Work out the finished part from the listing and answer in its coordinate system (mm). Coordinates: 2 decimals unless noted, no trailing zeros. Write each loop counter-clockwise with the first axis right and the second up, starting at its lowest first coordinate (ties: lowest second). Pieces come first, ordered by that corner, then holes. Notation, with made-up numbers: (17, 51) - (31, 51) arc R21 cw to (31, 63) - close; hole circle Ø9 at (86, -13). An arc over 180 degrees is marked (long way). Use a Markdown table: item, result. Add a question column.
(1) The part is cut by section A-A, the plane y = 22.5. Give the vertices of the cut face in (x, z), then the cut area to 3 significant figures.
(2) Given pin 1 Ø12 at (x, y) = (153, 104) entering from +Z; pin 2 Ø1 at (x, z) = (5.5, 1.5) entering from -Y; pin 3 Ø1 at (x, z) = (172, 1) entering from +Y; pin 4 Ø0.6 at (x, z) = (196, 1) entering from -Y, each flat-ended and moving along its own axis, determine where each tip first touches the part or whether it passes through.
(3) Find the intervals of material crossed by line 1 (X direction, y = 117, z = 0.25); line 2 (X direction, y = 87, z = 1.05); line 3 (X direction, y = 84, z = 1.2), in increasing order. Write a range as from..to.
(4) The part is cut by section B-B, the plane x = 110. Give the vertices of the cut face in (y, z), then the cut area to 3 significant figures.
from build123d import *

# Parameters (mm, degrees)
SKETCH1_W               = 194
SKETCH1_H               = 227
BOSS_EXTRUDE1_DEPTH     = 2
SKETCH2_W               = 2
SKETCH2_H               = 10
BOSS_EXTRUDE2_DEPTH     = 3
LPATTERN1_COUNT         = 11
LPATTERN1_PITCH         = 20
SKETCH4_W               = 2
SKETCH4_H               = 10
BOSS_EXTRUDE3_DEPTH     = 3
LPATTERN2_COUNT         = 11
LPATTERN2_PITCH         = 20
SKETCH5_W               = 10
SKETCH5_H               = 2
BOSS_EXTRUDE4_DEPTH     = 3
LPATTERN3_COUNT         = 9
LPATTERN3_PITCH         = 20
SKETCH6_W               = 10
SKETCH6_H               = 2
BOSS_EXTRUDE5_DEPTH     = 3
LPATTERN4_COUNT         = 9
LPATTERN4_PITCH         = 20
SKETCH7_W               = 30
SKETCH7_H               = 211
CUT_EXTRUDE1_DEPTH      = 3
SKETCH8_R               = 1.75
SKETCH8_W               = 30
SKETCH8_H               = 211
CUT_EXTRUDE2_DEPTH      = 3
ENL_V_START             = -2
ESQUISSE1_W             = 1
ESQUISSE1_H             = 231.630862985
ENL_V_MAT_EXTRU_1_DEPTH = 2
ESQUISSE2_W             = 1
ESQUISSE2_H             = 7
ESQUISSE2_H_2           = 10
ESQUISSE2_W_2           = 10
ESQUISSE2_H_3           = 1
ESQUISSE2_W_3           = 14
BOSS_EXTRU_1_DEPTH      = 2
ESQUISSE3_R             = 1.75
ENL_V_MAT_EXTRU_2_DEPTH = 3


with BuildPart() as part:
    # Sketch1 → Boss-Extrude1 (new body)
    with BuildSketch(Plane.XY):
        with Locations((97, 113.5)):
            Rectangle(SKETCH1_W, SKETCH1_H)
    extrude(amount=BOSS_EXTRUDE1_DEPTH)

    # Sketch2 → Boss-Extrude2 (add)
    with BuildSketch(Plane(origin=(194, 0, 0), x_dir=(0, 0, -1), z_dir=(1, 0, 0))):
        with Locations((-1, 15)):
            Rectangle(SKETCH2_W, SKETCH2_H)
    boss_extrude2 = extrude(amount=BOSS_EXTRUDE2_DEPTH)

    # LPattern1: Boss-Extrude2 ×11
    with Locations(*[(0, i * LPATTERN1_PITCH, 0) for i in range(1, LPATTERN1_COUNT)]):
        add(boss_extrude2)

    # Sketch4 → Boss-Extrude3 (add)
    with BuildSketch(Plane.ZY):
        with Locations((1, 15)):
            Rectangle(SKETCH4_W, SKETCH4_H)
    boss_extrude3 = extrude(amount=BOSS_EXTRUDE3_DEPTH)

    # LPattern2: Boss-Extrude3 ×11
    with Locations(*[(0, i * LPATTERN2_PITCH, 0) for i in range(1, LPATTERN2_COUNT)]):
        add(boss_extrude3)

    # Sketch5 → Boss-Extrude4 (add)
    with BuildSketch(Plane.XZ):
        with Locations((179, 1)):
            Rectangle(SKETCH5_W, SKETCH5_H)
    boss_extrude4 = extrude(amount=BOSS_EXTRUDE4_DEPTH)

    # LPattern3: Boss-Extrude4 ×9
    with Locations(*[(-i * LPATTERN3_PITCH, 0, 0) for i in range(1, LPATTERN3_COUNT)]):
        add(boss_extrude4)

    # Sketch6 → Boss-Extrude5 (add)
    with BuildSketch(Plane(origin=(0, 227, 0), x_dir=(1, 0, 0), z_dir=(0, 1, 0))):
        with Locations((179, -1)):
            Rectangle(SKETCH6_W, SKETCH6_H)
    boss_extrude5 = extrude(amount=BOSS_EXTRUDE5_DEPTH)

    # LPattern4: Boss-Extrude5 ×9
    with Locations(*[(-i * LPATTERN4_PITCH, 0, 0) for i in range(1, LPATTERN4_COUNT)]):
        add(boss_extrude5)

    # Sketch7 → Cut-Extrude1 (cut, through all)
    with BuildSketch(Plane.XY.offset(2)):
        with Locations((27, 113.5)):
            Rectangle(SKETCH7_W, SKETCH7_H)
    extrude(amount=-CUT_EXTRUDE1_DEPTH, mode=Mode.SUBTRACT)

    # Sketch8 → Cut-Extrude2 (cut, through all)
    with BuildSketch(Plane.XY.offset(2)):
        with Locations((143, 15)):
            Circle(SKETCH8_R)
        with Locations((51.5, 15)):
            Circle(SKETCH8_R)
        with Locations((143, 87)):
            Circle(SKETCH8_R)
        with Locations((51.5, 87)):
            Circle(SKETCH8_R)
        with Locations((134, 112)):
            Circle(SKETCH8_R)
        with Locations((76, 112)):
            Circle(SKETCH8_R)
        with Locations((134, 161)):
            Circle(SKETCH8_R)
        with Locations((76, 161)):
            Circle(SKETCH8_R)
        with Locations((167, 113.5)):
            Rectangle(SKETCH8_W, SKETCH8_H)
    extrude(amount=-CUT_EXTRUDE2_DEPTH, mode=Mode.SUBTRACT)

    # Esquisse1 → Enlèv. mat.-Extru.1 (cut)
    with BuildSketch(Plane(origin=(0, 0, 0), x_dir=(-1, 0, 0), z_dir=(0, 0, -1)).offset(ENL_V_START)):
        with Locations((2.5, 104.184568508)):
            Rectangle(ESQUISSE1_W, ESQUISSE1_H)
    extrude(amount=ENL_V_MAT_EXTRU_1_DEPTH, mode=Mode.SUBTRACT)

    # Esquisse2 → Boss.-Extru.1 (add)
    with BuildSketch(Plane(origin=(0, 0, 0), x_dir=(-1, 0, 0), z_dir=(0, 0, -1))):
        with Locations((-194.5, 223.5)):
            Rectangle(ESQUISSE2_W, ESQUISSE2_H)
        with Locations((-194.5, 205)):
            Rectangle(ESQUISSE2_W, ESQUISSE2_H_2)
        with Locations((-194.5, 185)):
            Rectangle(ESQUISSE2_W, ESQUISSE2_H_2)
        with Locations((-194.5, 165)):
            Rectangle(ESQUISSE2_W, ESQUISSE2_H_2)
        with Locations((-194.5, 145)):
            Rectangle(ESQUISSE2_W, ESQUISSE2_H_2)
        with Locations((-194.5, 125)):
            Rectangle(ESQUISSE2_W, ESQUISSE2_H_2)
        with Locations((-194.5, 105)):
            Rectangle(ESQUISSE2_W, ESQUISSE2_H_2)
        with Locations((-194.5, 85)):
            Rectangle(ESQUISSE2_W, ESQUISSE2_H_2)
        with Locations((-194.5, 65)):
            Rectangle(ESQUISSE2_W, ESQUISSE2_H_2)
        with Locations((-194.5, 45)):
            Rectangle(ESQUISSE2_W, ESQUISSE2_H_2)
        with Locations((-194.5, 25)):
            Rectangle(ESQUISSE2_W, ESQUISSE2_H_2)
        Polygon((-194, 0), (-194, 10), (-195, 10), (-195, -1), (-184, -1), (-184, 0), align=None)
        with Locations((-169, -0.5)):
            Rectangle(ESQUISSE2_W_2, ESQUISSE2_H_3)
        with Locations((-149, -0.5)):
            Rectangle(ESQUISSE2_W_2, ESQUISSE2_H_3)
        with Locations((-129, -0.5)):
            Rectangle(ESQUISSE2_W_2, ESQUISSE2_H_3)
        with Locations((-109, -0.5)):
            Rectangle(ESQUISSE2_W_2, ESQUISSE2_H_3)
        with Locations((-89, -0.5)):
            Rectangle(ESQUISSE2_W_2, ESQUISSE2_H_3)
        with Locations((-69, -0.5)):
            Rectangle(ESQUISSE2_W_2, ESQUISSE2_H_3)
        with Locations((-49, -0.5)):
            Rectangle(ESQUISSE2_W_2, ESQUISSE2_H_3)
        with Locations((-29, -0.5)):
            Rectangle(ESQUISSE2_W_2, ESQUISSE2_H_3)
        with Locations((-7, -0.5)):
            Rectangle(ESQUISSE2_W_3, ESQUISSE2_H_3)
    extrude(amount=-BOSS_EXTRU_1_DEPTH)

    # Esquisse3 → Enlèv. mat.-Extru.2 (cut, through all)
    with BuildSketch(Plane(origin=(0, 0, 0), x_dir=(-1, 0, 0), z_dir=(0, 0, -1))):
        with Locations((-96.112690171, 180.774445285)):
            Circle(ESQUISSE3_R)
        with Locations((-126.212690171, 131.674445285)):
            Circle(ESQUISSE3_R)
        with Locations((-83.112690171, 131.674445285)):
            Circle(ESQUISSE3_R)
    extrude(amount=-ENL_V_MAT_EXTRU_2_DEPTH, mode=Mode.SUBTRACT)


solid = part.part
Model answer:
| question | item | result |
|---|---|---|
| 1 | outline | (0, 0) - (12, 0) - (12, 2) - (0, 2) - close; (42, 0) - (152, 0) - (152, 2) - (42, 2) - close; (182, 0) - (195, 0) - (195, 2) - (182, 2) - close |
| 1 | area | 270 mm^2 |
| 2 | pin 1 | z = 2 |
| 2 | pin 2 | y = -1 |
| 2 | pin 3 | y = 227 |
| 2 | pin 4 | y = 10 |
| 3 | line 1 | -2..12, 42..152, 182..197 |
| 3 | line 2 | 0..12, 42..49.75, 53.25..141.25, 144.75..152, 182..195 |
| 3 | line 3 | 0..12, 42..152, 182..195 |
| 4 | outline | (-1, 0) - (227, 0) - (227, 2) - (-1, 2) - close |
| 4 | area | 456 mm^2 |
